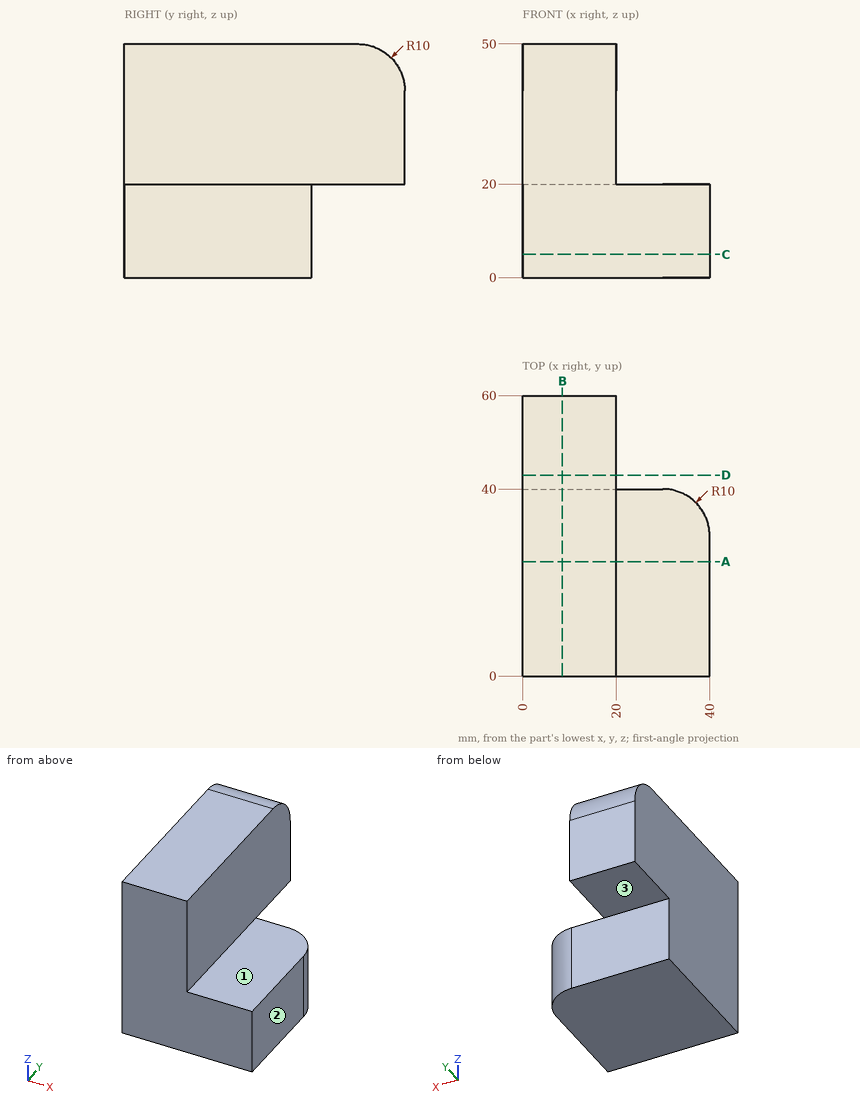
Geometry check sheet. Reference: drawing and pictorial views, mm from the part's lowest x, y, z. A direction names the side the tool comes from. Give positions to 0.01 mm unless a question says otherwise; leave off trailing zeros. Order: outer loops, then holes, each group sorted by start corner. A loop starts at its lowest first (then second) coordinate and runs counter-clockwise, first axis right, second up. Notation, with made-up numbers: M -29.75,25.25 L 24.25,25.25 A30 ccw 24.25,50.25 Z; hole C -14,79 d7. An arc over 180 degrees is marked long. Answer in a Markdown table with one row per item.
1) Gauge pin test, flat ends, axial feed: P1, Ø12, axis at x = 19.5, z = 31, coming from the -Y side; P2, Ø16, axis at x = 32.5, y = 17, coming from the +Z side; P3, Ø3, axis at x = 20, z = 13, coming from the +Y side; P4, Ø1.5, axis at y = 19, z = 21.5, coming from the +X side. Record the tip position at first contact, or that the pin passes through.
Filled sheet:
| item | result |
|---|---|
| P1 | stops at y = 0 |
| P2 | stops at z = 20 |
| P3 | stops at y = 40 |
| P4 | stops at x = 20 |
2) Thickness scan on L1, parallel to X at y = 10, z = 45; L2, parallel to Y at x = 20.5, z = 8.5. Record the ranges inside material, lowest first. Write a range as [from, to].
Filled sheet:
| item | result |
|---|---|
| L1 | x = [0, 20] |
| L2 | y = [0, 40] |
3) Access from +Z, -Z, +X, -X, +Y, -Y to the whole of each face (thin tool, end or side, straight path). Record for the marked faces 1, 2 and 3.
Filled sheet:
| item | result |
|---|---|
| face 1 | +Z, +X, +Y, -Y |
| face 2 | +Z, -Z, +X, +Y, -Y |
| face 3 | -Z, +X, -X, +Y |
4) Cross-section at D-D, the plane y = 43. Enter the section's corners in (x, z), plus the area to 3 significant figures.
Filled sheet:
| item | result |
|---|---|
| outline | M 0,20 L 20,20 L 20,50 L 0,50 Z |
| area | 600 mm2 |
5) Cross-section at B-B, the plane x = 8.5. Enter the section's corners in (y, z), plus the area to 3 significant figures.
Filled sheet:
| item | result |
|---|---|
| outline | M 0,0 L 40,0 L 40,20 L 60,20 L 60,40 A10 ccw 50,50 L 0,50 Z |
| area | 2,580 mm2 |
6) Cross-section at C-C, the plane z = 5. Enter the section's corners in (x, y), plus the area to 3 significant figures.
Filled sheet:
| item | result |
|---|---|
| outline | M 0,0 L 40,0 L 40,30 A10 ccw 30,40 L 0,40 Z |
| area | 1,580 mm2 |
7) Cross-section at A-A, the plane y = 24.5. Enter the section's corners in (x, z), plus the area to 3 significant figures.
Filled sheet:
| item | result |
|---|---|
| outline | M 0,0 L 40,0 L 40,20 L 20,20 L 20,50 L 0,50 Z |
| area | 1,400 mm2 |
